Autodesk Inventor part; units mm, degrees
ref_plane "YZ Plane" through (0, 0, 0) normal (1, 0, 0) x (0, 1, 0)
ref_plane "XZ Plane" through (0, 0, 0) normal (0, 1, 0) x (-1, 0, 0)
ref_plane "XY Plane" through (0, 0, 0) normal (0, 0, 1) x (1, 0, 0)
sketch "Boceto3" plane through (0, 0, 0) normal (0, 1, 0) x (-1, 0, 0)
  line L0 (-109, -180) -> (109, -180)
  line L1 (109, -180) -> (109, 180)
  line L2 (109, 180) -> (-109, 180)
  line L3 (-109, 180) -> (-109, -180)
  line L4 (-109, -180) -> (109, 180) construction
  line L5 (109, -180) -> (-109, 180) construction
  line L6 (0, 180) -> (103.5, 180)
  line L7 (109, 180) -> (97.75, 180)
  line L8 (97.75, 180) -> (97.75, 160)
  line L9 (97.75, 180) -> (117.75, 180) construction
  line L10 (97.75, 160) -> (105.25, 160)
  line L11 (105.25, 160) -> (105.25, 145)
  line L12 (105.25, 145) -> (97.75, 145)
  line L13 (97.75, 145) -> (97.75, 142)
  line L14 (97.75, 142) -> (109, 142)
  line L15 (109, -180) -> (97.75, -180)
  line L16 (97.75, -180) -> (97.75, -160)
  line L17 (97.75, -180) -> (117.75, -180) construction
  line L18 (97.75, -160) -> (105.25, -160)
  line L19 (105.25, -160) -> (105.25, -145)
  line L20 (105.25, -145) -> (97.75, -145)
  line L21 (97.75, -145) -> (97.75, -142)
  line L22 (97.75, -142) -> (109, -142)
  line L23 (-109, 180) -> (-102.7, 180)
  line L24 (-109, 180) -> (-109, 160)
  line L25 (-109, 160) -> (-115.3, 160)
  line L26 (-109, 160) -> (-109, 146.9)
  line L27 (-115.3, 146.9) -> (-109, 146.9)
  line L28 (-109, 146.9) -> (-109, -180)
  line L29 (-102.7, -180) -> (-102.7, -160)
  line L30 (-102.7, -180) -> (-82.7, -180) construction
  line L31 (-109, -160) -> (-115.3, -160)
  line L32 (-109, -160) -> (-109, -146.9)
  line L33 (-115.3, -146.9) -> (-109, -146.9)
  line L34 (-115.3, 160) -> (-115.3, 146.9)
  line L35 (-115.3, -146.9) -> (-115.3, -160)
  point P0 (0, 0)
  point P1 (-109, -180)
  dimension "d27" = 218
  dimension "d28" = 360
  dimension "d33" = 11.25
  dimension "d34" = 20
  dimension "d35" = 90
  dimension "d36" = 7.5
  dimension "d37" = 15
  dimension "d38" = 7.5
  dimension "d39" = 3
  dimension "d40" = 11.25
  dimension "d41" = 20
  dimension "d42" = 90
  dimension "d43" = 15
  dimension "d44" = 3
  dimension "d45" = 6.3
  dimension "d46" = 20
  dimension "d47" = 90
  dimension "d48" = 13.1
  dimension "d49" = 90
  dimension "d50" = 20
  dimension "d51" = 90
  dimension "d52" = 13.1
extrude "Extrusión2" add sketch "Boceto3" along normal blind 3.6 contours L3 L2 L8 L10 L11 L12 L13 L14 L1 L22 L21 L20 L19 L18 L16 L0 | L31 L35 L33 L3 | L27 L34 L25 L3
sketch "Boceto4" plane through (0, 3.6, 0) normal (0, 1, 0) x (1, 0, 0)
  line L0 (-105.25, -145) -> (-105.25, -160)
  line L1 (-105.25, -160) -> (-97.75, -160)
  line L2 (-97.75, -145) -> (-105.25, -145)
  point P0 (0, 0)
  point P1 (-100.65, -156.7)
  point P2 (-100.65, -148.3)
  dimension "d55" = 4.6
  dimension "d56" = 3.3
  dimension "d73" = 3.3
  dimension "d74" = 4.6
hole "Agujero1" at (-100.65, 3.6, 156.7) at (-100.65, 3.6, 148.3) direction (0, -1, 0) diameter 3.3 end through all
mirror "Simetría1" about plane through (0, 0, 0) normal (0, 0, 1) of "Agujero1"
sketch "Boceto6" plane through (0, 3.6, 0) normal (0, 1, 0) x (1, 0, 0)
  line L0 (109, -160) -> (115.3, -160)
  line L1 (109, 160) -> (109, 180)
  line L2 (115.3, -146.9) -> (109, -146.9)
  line L3 (115.3, -156.3) -> (111.9, -156.3)
  line L4 (111.9, -156.3) -> (111.9, -150.6)
  circle A0 centre (111.9, -156.3) radius 1.2
  circle A1 centre (111.9, -150.6) radius 1.2
  point P0 (0, 0)
  point P1 (105.6, -156.3)
  point P2 (102.7, -160)
  point P3 (105.6, -150.6)
  point P4 (102.7, -146.9)
  dimension "d75" = 3.7
  dimension "d76" = 3.4
  dimension "d77" = 3.7
  dimension "d78" = 3.4
  dimension "d95" = 3.4
  dimension "d96" = 2.4
  dimension "d97" = 2.4
hole "Agujero3" at (111.9, 3.6, 156.3) at (111.9, 3.6, 150.6) direction (0, -1, 0) diameter 2.4 end through all
mirror "Simetría2" about plane through (0, 0, 0) normal (0, 0, 1) of "Agujero3"
equation "\"d57\" = d73"
properties part number "pantalla"
Check sheet for the modelled part. Datum: model origin and axes. Units: mm. Coordinates: 2 decimals unless noted, no trailing zeros. Loops run counter-clockwise (first coordinate to the right, second up) from the corner with the lowest first, then second, coordinate; pieces in that order, holes last.
1) Sectioned sample at A-A (y = 2.15). Count the separate pieces of the cut face and the enclosed holes in it, and give its area (3 significant figures).
2) Sectioned sample at B-B (z = -119.5). Record the boundary of the cut face in (x, y), and give its area (3 significant figures).
3) Gauge pin test, flat ends, axial feed: pin 1 (4 mm diameter, centred on x = -100.65, z = -148.3, fed in from +Y); pin 2 (1.1 mm diameter, centred on y = 2.5, z = 156, fed in from -X); pin 3 (1.8 mm diameter, centred on x = -100.5, y = 2.5, fed in from +Z); pin 4 (3 mm diameter, centred on x = -100.65, z = -156.7, fed in from +Y). Record the tip position at first contact, or that the pin passes through.
4) Material ranges on probe 1 along Z at (x, y) = (111.9, 2.55); probe 2 along X at (y, z) = (0.95, -156.7); probe 3 along X at (y, z) = (2, 156.3), recorded low to high.
Check sheet entries:
1. separate pieces: 1
1. enclosed holes: 8
1. area: 78,000 mm2
2. outline: (-109, 0) - (109, 0) - (109, 3.6) - (-109, 3.6) - close
2. area: 785 mm2
3. pin 1: stops at y = 3.6
3. pin 2: stops at x = -105.25
3. pin 3: stops at z = 160
3. pin 4: passes through
4. probe 1: z = -160 to -157.5, -155.1 to -151.8, -149.4 to -146.9, 146.9 to 149.4, 151.8 to 155.1, 157.5 to 160
4. probe 2: x = -105.25 to -102.3, -99 to 110.77, 113.03 to 115.3
4. probe 3: x = -105.25 to -102.25, -99.05 to 110.7, 113.1 to 115.3
